Source: three-view drawing plus pictorial views. Frame: mm from the lowest corner of the part. A direction names the side the tool comes from. Coordinates: 2 decimals unless noted, no trailing zeros. Write each loop counter-clockwise with the first axis right and the second up, starting at its lowest first coordinate (ties: lowest second). Pieces come first, ordered by that corner, then holes. Notation, with made-up numbers: (-18.75, 23.5) -> (-14.75, 23.5) arc R14 cw to (-14.75, 46.5) -> close; hole circle Ø6 at (18.25, -4.75). An arc over 180 degrees is marked (long way). One line per item, written item: value. Start each with the question number.
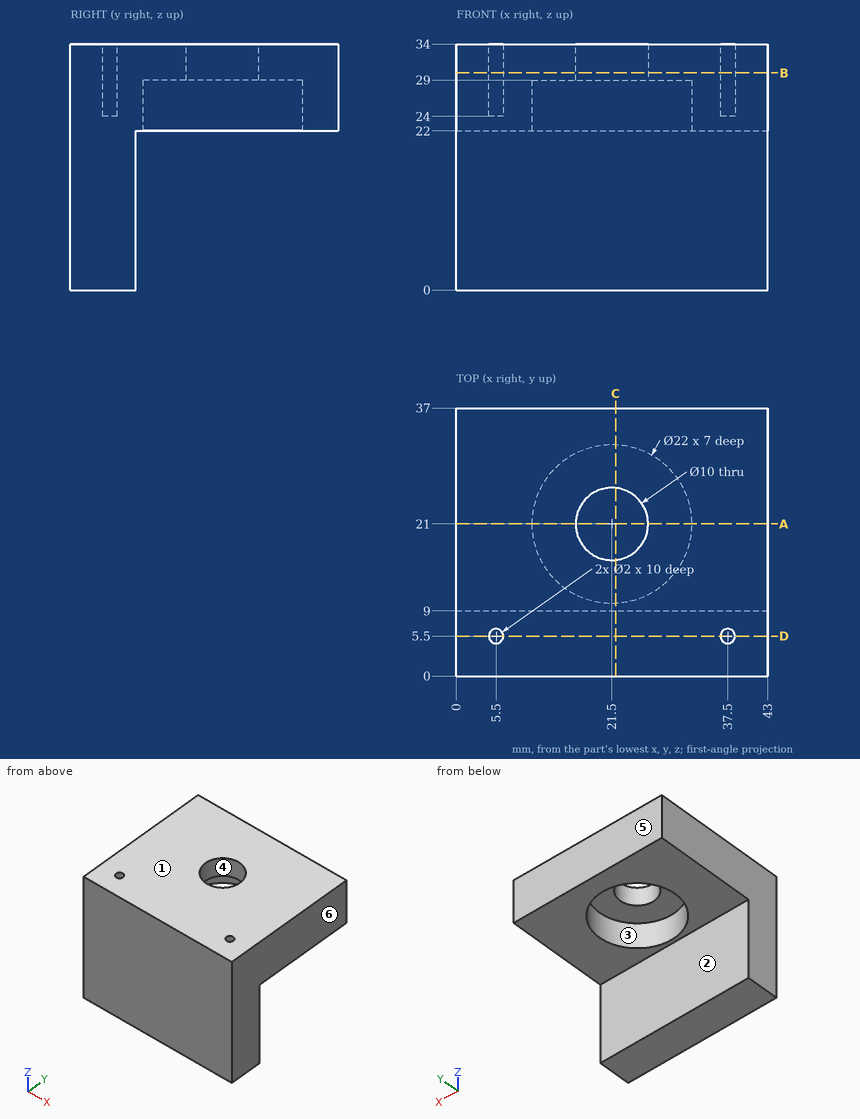
Q1. First-contact query: P1, Ø2, axis at x = 15.5, z = 16.5, coming from the +Y side; P2, Ø6.5, axis at x = 25.5, y = 20.5, coming from the -Z side; P3, Ø1.2, axis at x = 37.5, y = 5.5, coming from the +Z side; P4, Ø12, axis at y = 28.5, z = 13, coming from the -X side. Flat tips, straight axial feed; report the tip coordinate or a pass-through.
Q2. Line query: L1, parallel to Y at x = 21.5, z = 31.05; L2, parallel to Y at x = 21.5, z = 27; L3, parallel to X at y = 5, z = 32. Output: solid intervals per line, ascending. Write a range as from..to.
Q3. Cut plane A-A on y = 21. Output: boundary loops of the cut face in (x, z).
Q4. Access query for the marked faces 1, 2 and 3. Directions: +Z, -Z, +X, -X, +Y, -Y. A direction counts if a zero-diameter tool reaches every point of the face in a straight line with its end or side. Return the directions, or none.
Q5. Draft query along Y for the marked faces 4, 5 and 6. Return one class per face: pulls with the +Y half, pulls with the -Y half, needs draft (parallel to the pull), parting line crosses it, or undercut.
Q6. Cut plane C-C on x = 22. Output: boundary loops of the cut face in (y, z), and give its area (3 significant figures).
Q7. Cut plane D-D on y = 5.5. Output: boundary loops of the cut face in (x, z), and give its area (3 significant figures).
Q8. Cut plane B-B on z = 30. Output: boundary loops of the cut face in (x, y), and give its area (3 significant figures).
Solution:
1. P1: y = 9
1. P2: z = 29
1. P3: z = 24
1. P4: through
2. L1: 0..16, 26..37
2. L2: 0..10, 32..37
2. L3: 0..4.63, 6.37..36.63, 38.37..43
3. outline: (0, 22) -> (10.5, 22) -> (10.5, 29) -> (16.5, 29) -> (16.5, 34) -> (0, 34) -> close; (26.5, 29) -> (32.5, 29) -> (32.5, 22) -> (43, 22) -> (43, 34) -> (26.5, 34) -> close
4. face 1: +Z, +X, -X, +Y, -Y
4. face 2: -Z, +X, -X, +Y
4. face 3: -Z
5. face 4: undercut
5. face 5: pulls with the +Y half
5. face 6: needs draft
6. outline: (0, 0) -> (9, 0) -> (9, 22) -> (10.01, 22) -> (10.01, 29) -> (16.03, 29) -> (16.03, 34) -> (0, 34) -> close; (25.97, 29) -> (31.99, 29) -> (31.99, 22) -> (37, 22) -> (37, 34) -> (25.97, 34) -> close
6. area: 438 mm²
7. outline: (0, 0) -> (43, 0) -> (43, 34) -> (38.5, 34) -> (38.5, 24) -> (36.5, 24) -> (36.5, 34) -> (6.5, 34) -> (6.5, 24) -> (4.5, 24) -> (4.5, 34) -> (0, 34) -> close
7. area: 1,420 mm²
8. outline: (0, 0) -> (43, 0) -> (43, 37) -> (0, 37) -> close; hole circle Ø2 at (5.5, 5.5); hole circle Ø10 at (21.5, 21); hole circle Ø2 at (37.5, 5.5)
8. area: 1,510 mm²
